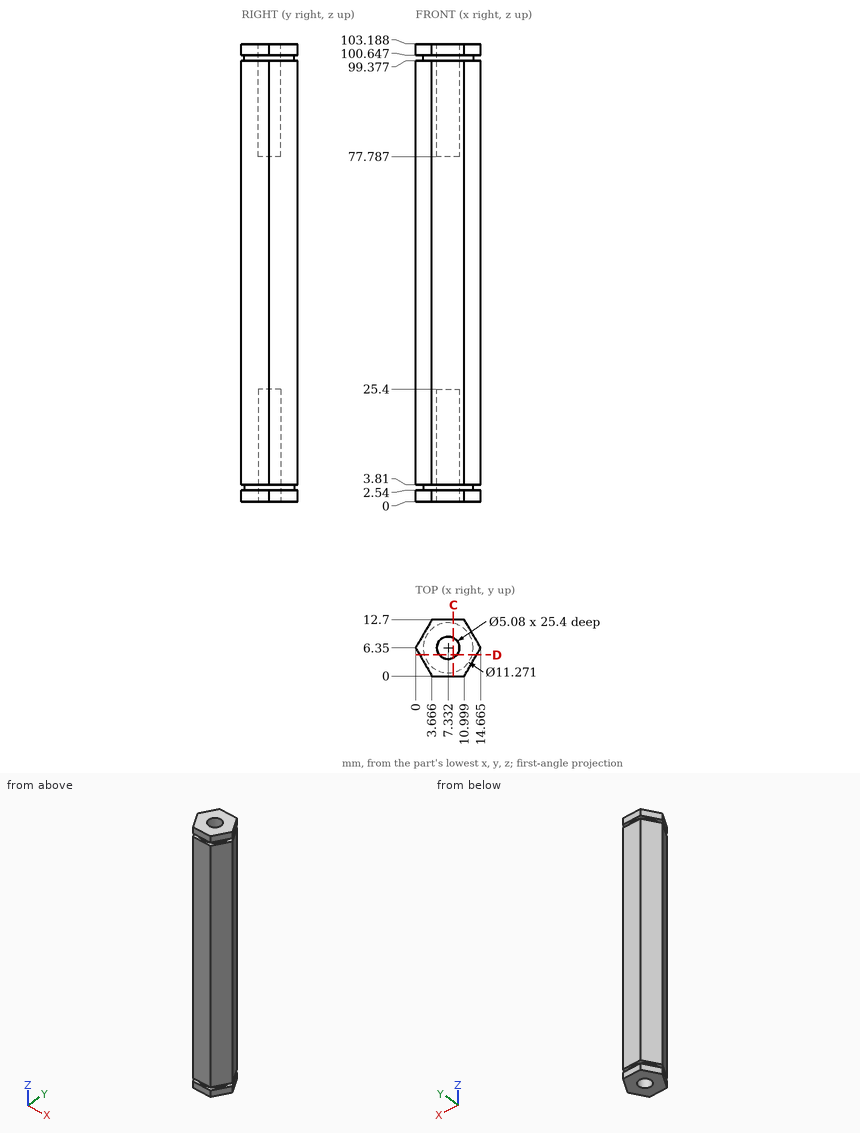
Can you work these out from the drawing? Everything is in mm from the part's minimum corner. Give positions to 0.01 mm unless a question says otherwise; leave off trailing zeros. Order: outer loops, then holes, each group sorted by start corner. A loop starts at its lowest first (then second) coordinate and runs counter-clockwise, first axis right, second up. Notation, with made-up numbers: M -7,65.5 L 36,65.5 A28 cw 36,96.5 Z; hole C 5,50 d4. An arc over 180 degrees is marked long. One line per question, with ' | ' between items.
1. I want a section at C-C (x = 8.5). List the corners of the cut face in (y, z) for me (1 decimal), and give its area (3 significant figures).
Results:
outline: M 0,0 L 4.1,0 L 4.1,25.4 L 8.6,25.4 L 8.6,0 L 12.7,0 L 12.7,2.5 L 11.9,2.5 L 11.9,3.8 L 12.7,3.8 L 12.7,99.4 L 11.9,99.4 L 11.9,100.6 L 12.7,100.6 L 12.7,103.2 L 8.6,103.2 L 8.6,77.8 L 4.1,77.8 L 4.1,103.2 L 0,103.2 L 0,100.6 L 0.8,100.6 L 0.8,99.4 L 0,99.4 L 0,3.8 L 0.8,3.8 L 0.8,2.5 L 0,2.5 Z | area: 1,080 mm²
2. If I drill on line 1 (Z direction, x = 11.25, y = 1.75); line 2 (X direction, y = 7, z = 89) (1 decimal); line 3 (Z direction, x = 6, y = 5.5), over which ranges is the centre line in solid material (lowest first)?
Results:
line 1: 0 to 2.54, 3.81 to 99.38, 100.65 to 103.19 | line 2: 0.4 to 4.9, 9.8 to 14.3 | line 3: 25.4 to 77.79
3. I'm going to push flat-ended pins straight in: pin 1 (4 mm diameter, centred on y = 9, z = 12, fed in from -X) (1 decimal); pin 2 (1.5 mm diameter, centred on x = 8, y = 6, fed in from -Z); pin 3 (1.5 mm diameter, centred on x = 6.5, y = 7.5, fed in from +Z). Where does each tip first touch, or does it pass through?
Results:
pin 1: x = 0.4 | pin 2: z = 25.4 | pin 3: z = 77.79
4. I want a section at D-D (y = 4.75). List the corners of the cut face in (x, z) for me (1 decimal).
Results:
outline: M 0.9,0 L 5.4,0 L 5.4,25.4 L 9.3,25.4 L 9.3,0 L 13.7,0 L 13.7,2.5 L 12.7,2.5 L 12.7,3.8 L 13.7,3.8 L 13.7,99.4 L 12.7,99.4 L 12.7,100.6 L 13.7,100.6 L 13.7,103.2 L 9.3,103.2 L 9.3,77.8 L 5.4,77.8 L 5.4,103.2 L 0.9,103.2 L 0.9,100.6 L 1.9,100.6 L 1.9,99.4 L 0.9,99.4 L 0.9,3.8 L 1.9,3.8 L 1.9,2.5 L 0.9,2.5 Z
